Here's the drawing with two shaded views (mm, measured from the low corner). I have some questions. A direction names the side the tool comes from. Coordinates: 2 decimals unless noted, no trailing zeros. Loops run counter-clockwise (first coordinate to the right, second up) from the corner with the lowest first, then second, coordinate; pieces in that order, holes last.
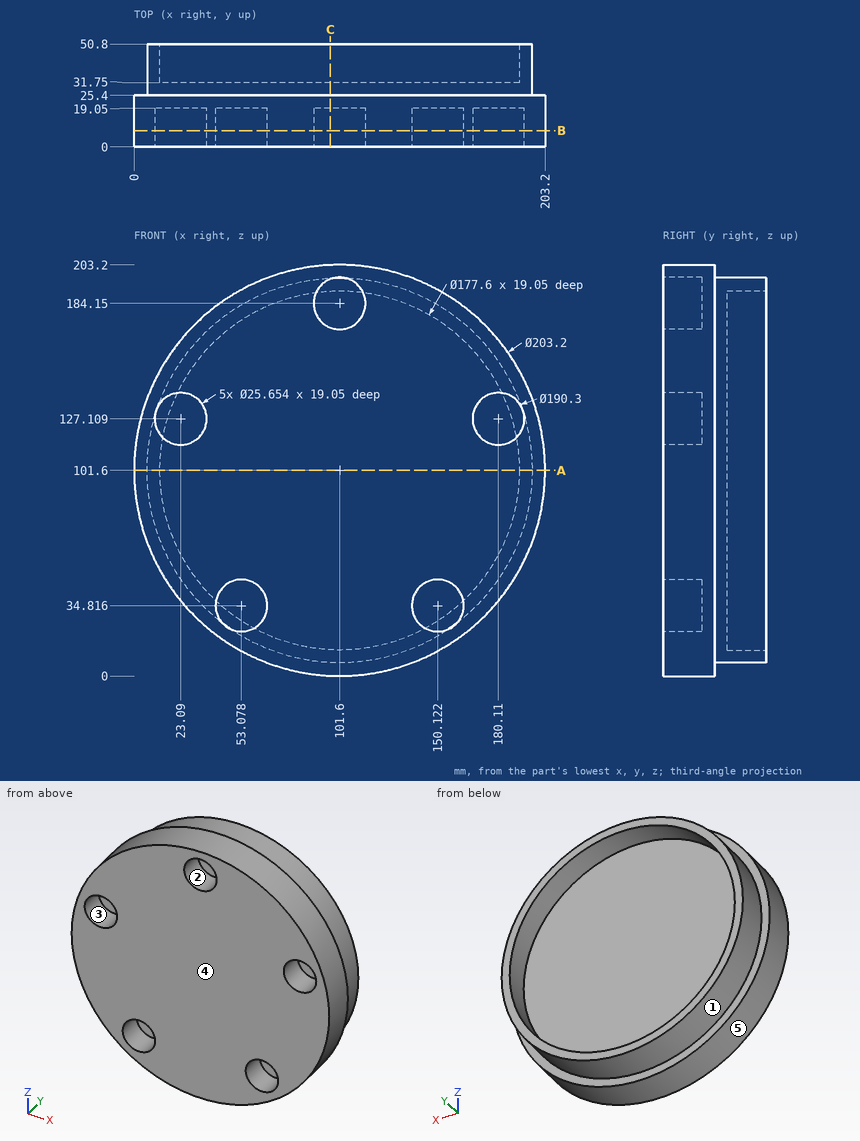
Q1. Please list where these lines run through material, in increasing order: probe 1 along Z at (x, y) = (101.6, 40.5); probe 2 along Z at (x, y) = (101.6, 11.25).
Q2. We'd pull the mould along X, two halves only. Please class the marked faces 3, 4 and 5: pulls with the +X half, pulls with the -X half, needs draft (parallel to the pull), parting line crosses it, or undercut.
Q3. For the marked faces 1 and 2, which set-ups out of +Z, -Z, +X, -X, +Y, -Y let a thin tool reach every point of the face, with its end or its side?
Q4. Suppose I cut it at C-C on x = 97. Write out the boundary of the cut face in (y, z).
Q5. Suppose I cut it at A-A on z = 101.6. Write out the boundary of the cut face in (x, y), and give its area (3 significant figures).
Q6. Suppose I cut it at B-B on y = 8. State how many separate pieces and enclosed holes the cut face has, and give its area (3 significant figures).
Q7. Will these pins go through, and if not, where does the flat tip stop? P1, Ø13, axis at x = 145, z = 36, coming from the -Y side; P2, Ø5, axis at x = 137.5, y = 29.5, coming from the +Z side (1 decimal); P3, Ø1, axis at x = 97, y = 30, coming from the +Z side.
Check values:
1. probe 1: z = 6.45 to 12.8, 190.4 to 196.75
1. probe 2: z = 0 to 171.32, 196.98 to 203.2
2. face 3: undercut
2. face 4: needs draft
2. face 5: parting line crosses it
3. face 1: +Y
3. face 2: -Y
4. outline: (0, 0.1) - (25.4, 0.1) - (25.4, 6.56) - (50.8, 6.56) - (50.8, 12.92) - (31.75, 12.92) - (31.75, 190.28) - (50.8, 190.28) - (50.8, 196.64) - (25.4, 196.64) - (25.4, 203.1) - (0, 203.1) - (0, 196.12) - (19.05, 196.12) - (19.05, 172.18) - (0, 172.18) - close
5. outline: (0, 0) - (203.2, 0) - (203.2, 25.4) - (196.75, 25.4) - (196.75, 50.8) - (190.4, 50.8) - (190.4, 31.75) - (12.8, 31.75) - (12.8, 50.8) - (6.45, 50.8) - (6.45, 25.4) - (0, 25.4) - close
5. area: 6,610 mm2
6. separate pieces: 1
6. enclosed holes: 5
6. area: 29,800 mm2
7. P1: stops at y = 19.05
7. P2: stops at z = 190.7
7. P3: stops at z = 196.66
